The model under review builds one solid part; all positions refer to its coordinate system, in mm. A direction names the side the tool comes from. Give positions to 0.01 mm unless a question says otherwise; leave off trailing zeros. Loops run counter-clockwise (first coordinate to the right, second up) from the corner with the lowest first, then second, coordinate; pieces in that order, holes last. Notation, with made-up numbers: M 1.5,39 L 33.5,39 A13 ccw 33.5,63 Z; hole C 4.25,6 d1. An arc over 180 degrees is marked long. Write item = value, one per line. Start each with the question number.
1. We need section B-B on z = -9. Give the boundary of the cut face in (x, y).
2. We need section D-D on x = 16.5. Give the boundary of the cut face in (y, z), then the cut area to 3 significant figures.
3. Wall thickness on line 1 along Y through (x, z) = (-5.5, -9): over which ranges is the line inside the solid? List them lowest first. Write a range as from..to.
4. For faces 1 (the face through (4, -18, 9.61)), 2 (the face through (2.83, -41.93, -2.21)), list the 3-axis set-ups (+Z, -Z, +X, -X, +Y, -Y) from which the entire face can be reached by the end or side of a thin tool; tool diameter is ignored.
5. We need section C-C on y = -39. Give the boundary of the cut face in (x, z).
6. We need section A-A on x = 3. Give the boundary of the cut face in (y, z).
7. For pin 1 (6.5 mm diameter, centred on x = 9.5, z = 4.5, fed in from -Y), flat-tipped, find the tip position at first contact; note if it passes through.
from build123d import *

# Parameters (mm, degrees)
F0_W     = 30
F0_H     = 21
F1_DEPTH = 37
F2_W     = 5
F2_H     = 5
F3_DEPTH = 37
F4_R     = 1.5
F5_DEPTH = 10


with BuildPart() as f1:
    # F0 (on Front) → F1 (new body)
    with BuildSketch(Plane.XZ):
        with Locations((4.018988, -0.890413)):
            Rectangle(F0_W, F0_H)
    extrude(amount=F1_DEPTH)

    # F2 (on face) → F3 (join)
    with BuildSketch(Plane(origin=(0, 0, 0), x_dir=(-1, 0, 0), z_dir=(0, 1, 0))):
        with Locations((-16.518988, -8.890413)):
            Rectangle(F2_W, F2_H)
    extrude(amount=-F3_DEPTH)

    # F4 (on face) → F5 (join)
    with BuildSketch(Plane.XZ.offset(37)):
        with Locations((4.018988, -1.295996)):
            Circle(F4_R)
    extrude(amount=F5_DEPTH)


solid = f1.part
Final values:
q1.outline = M -10.98,-37 L 19.02,-37 L 19.02,0 L -10.98,0 Z
q2.outline = M -37,-11.39 L 0,-11.39 L 0,9.61 L -37,9.61 Z
q2.area = 777 mm²
q3.line_1 = -37..0
q4.face_1 = +Z, +X, -X, +Y, -Y
q4.face_2 = -Y
q5.outline = C 4.02,-1.3 d3
q6.outline = M -47,-2.4 L -37,-2.4 L -37,-11.39 L 0,-11.39 L 0,9.61 L -37,9.61 L -37,-0.2 L -47,-0.2 Z
q7.pin_1 = -37
